```python
from build123d import *

# Parameters (mm, degrees)
SKETCH1_W           = 100
SKETCH1_H           = 45
BOSS_EXTRUDE1_DEPTH = 21
CUT_EXTRUDE1_DEPTH  = 105.629106849
CUT_EXTRUDE2_DEPTH  = 10
CUT_EXTRUDE3_DEPTH  = 57.127087934
SKETCH6_R           = 3
CUT_EXTRUDE4_DEPTH  = 56.921820428
FILLET1_R           = 4.5
SKETCH7_R           = 18
CUT_EXTRUDE5_DEPTH  = 2


with BuildPart() as part:
    # Sketch1 → Boss-Extrude1 (new body)
    with BuildSketch(Plane(origin=(0, 0, 0), x_dir=(1, 0, 0), z_dir=(0, 1, 0))):
        Rectangle(SKETCH1_W, SKETCH1_H)
    extrude(amount=BOSS_EXTRUDE1_DEPTH)

    # Sketch2 → Cut-Extrude1 (cut, through all)
    with BuildSketch(Plane(origin=(50, 0, 0), x_dir=(0, 0, -1), z_dir=(1, 0, 0))):
        Polygon((-22.5, 0), (-22.5, 5), (-15.5, 0), align=None)
        Polygon((22.5, 0), (15.5, 0), (22.5, 5), align=None)
    extrude(amount=-CUT_EXTRUDE1_DEPTH, mode=Mode.SUBTRACT)

    # Sketch3 → Cut-Extrude2 (cut)
    with BuildSketch(Plane(origin=(0, 21, 0), x_dir=(1, 0, 0), z_dir=(0, 1, 0))):
        with BuildLine():
            Line((-42, 22.5), (-42, 18))
            ThreePointArc((-42, 18), (-43.025126266, 15.525126266), (-45.5, 14.5))
            Line((-45.5, 14.5), (-50, 14.5))
            Line((-50, 14.5), (-50, 22.5))
            Line((-50, 22.5), (-42, 22.5))
        make_face()
        with BuildLine():
            Line((-50, -22.5), (-42, -22.5))
            Line((-42, -22.5), (-42, -18))
            ThreePointArc((-42, -18), (-43.025126266, -15.525126266), (-45.5, -14.5))
            Line((-45.5, -14.5), (-50, -14.5))
            Line((-50, -14.5), (-50, -22.5))
        make_face()
        with BuildLine():
            Line((42, -22.5), (42, -18))
            ThreePointArc((42, -18), (43.025126266, -15.525126266), (45.5, -14.5))
            Line((45.5, -14.5), (50, -14.5))
            Line((50, -14.5), (50, -22.5))
            Line((50, -22.5), (42, -22.5))
        make_face()
        with BuildLine():
            Line((50, 22.5), (42, 22.5))
            Line((42, 22.5), (42, 18))
            ThreePointArc((42, 18), (43.025126266, 15.525126266), (45.5, 14.5))
            Line((45.5, 14.5), (50, 14.5))
            Line((50, 14.5), (50, 22.5))
        make_face()
    extrude(amount=-CUT_EXTRUDE2_DEPTH, mode=Mode.SUBTRACT)

    # Sketch5 → Cut-Extrude3 (cut, through all)
    with BuildSketch(Plane(origin=(0, 9, 0), x_dir=(1, 0, 0), z_dir=(0, 1, 0))):
        with BuildLine():
            Line((-45.5, -14.5), (-50, -14.5))
            Line((-50, -14.5), (-50, -22.5))
            Line((-50, -22.5), (-42, -22.5))
            Line((-42, -22.5), (-42, -18))
            ThreePointArc((-42, -18), (-43.025126266, -15.525126266), (-45.5, -14.5))
        make_face()
        with BuildLine():
            Line((42, -18), (42, -22.5))
            Line((42, -22.5), (50, -22.5))
            Line((50, -22.5), (50, -14.5))
            Line((50, -14.5), (45.5, -14.5))
            ThreePointArc((45.5, -14.5), (43.025126266, -15.525126266), (42, -18))
        make_face()
        with BuildLine():
            Line((45.5, 14.5), (50, 14.5))
            Line((50, 14.5), (50, 22.5))
            Line((50, 22.5), (42, 22.5))
            Line((42, 22.5), (42, 18))
            ThreePointArc((42, 18), (43.025126266, 15.525126266), (45.5, 14.5))
        make_face()
        with BuildLine():
            Line((-42, 22.5), (-50, 22.5))
            Line((-50, 22.5), (-50, 14.5))
            Line((-50, 14.5), (-45.5, 14.5))
            ThreePointArc((-45.5, 14.5), (-43.025126266, 15.525126266), (-42, 18))
            Line((-42, 18), (-42, 22.5))
        make_face()
    extrude(amount=-CUT_EXTRUDE3_DEPTH, mode=Mode.SUBTRACT)

    # Sketch6 → Cut-Extrude4 (cut, through all)
    with BuildSketch(Plane(origin=(0, 11, 0), x_dir=(1, 0, 0), z_dir=(0, 1, 0))):
        with Locations(Location((-45.5, 18, 0), (0, 0, 270))):
            Circle(SKETCH6_R)
        with Locations(Location((-45.5, -18, 0), (0, 0, 270))):
            Circle(SKETCH6_R)
        with Locations(Location((45.5, -18, 0), (0, 0, 270))):
            Circle(SKETCH6_R)
        with Locations(Location((45.5, 18, 0), (0, 0, 270))):
            Circle(SKETCH6_R)
    extrude(amount=-CUT_EXTRUDE4_DEPTH, mode=Mode.SUBTRACT)

    # Fillet1
    fillet1_edges = [part.edges().sort_by_distance(p)[0] for p in [
        (-50, 10, 22.5),
        (50, 10, 22.5),
        (-50, 10, -22.5),
        (50, 10, -22.5),
    ]]
    fillet(fillet1_edges, radius=FILLET1_R)

    # Sketch7 → Cut-Extrude5 (cut)
    with BuildSketch(Plane(origin=(0, 21, 0), x_dir=(1, 0, 0), z_dir=(0, 1, 0))):
        with Locations(Location((-21, 0, 0), (0, 0, 270))):
            Circle(SKETCH7_R)
        with Locations(Location((21, 0, 0), (0, 0, 270))):
            Circle(SKETCH7_R)
    extrude(amount=-CUT_EXTRUDE5_DEPTH, mode=Mode.SUBTRACT)


solid = part.part
```
CAD build for the part. Positions are in the model's coordinates, mm. A direction names the side the tool comes from. Round coordinates to 2 decimals unless told otherwise and drop trailing zeros. Loops run counter-clockwise (first coordinate to the right, second up) from the corner with the lowest first, then second, coordinate; pieces in that order, holes last. Notation, with made-up numbers: M -11,-15 L 47,-15 A22 ccw 47,23 Z; hole C 56,21 d4. An arc over 180 degrees is marked long. Return JSON: item names as keys, results as strings. Group by question number.
(1) Drop flat-ended pins along their axis: P1, Ø1.3, axis at x = 47.5, y = 16, coming from the -Z side; P2, Ø5, axis at x = 47, y = 16, coming from the +Z side; P3, Ø1.3, axis at x = -48.5, y = 16.5, coming from the +Z side; P4, Ø2.5, axis at x = 47, z = 18.5, coming from the +Y side. Give the stop position or say it passes through.
(2) Saw through at A-A, the plane y = 3.25. List the corners of the cut face in (x, z), and give its area (3 significant figures).
(3) Tool access for faces 1 (the flat face through (48, 16, -14.5)), 2 (the flat face through (48, 5, -14.5)), 3 (the cylindrical face through (-31.953, 20.014, -14.284)), 4 (the flat face through (-48, 9, -20)): list every direction of +Z, -Z, +X, -X, +Y, -Y with a clear straight run to the whole face (end or side of a thin tool).
(4) Wall check: probe 1 along X at (y, z) = (10.3, 18); probe 2 along X at (y, z) = (14, 15.5); probe 3 along X at (y, z) = (2.25, 18.5). Give the ranges that are in metal, low to high. Write a range as [from, to].
(5) Saw through at B-B, the plane z = -17. List the corners of the cut face in (x, y), and give its area (3 significant figures).
(6) Saw through at D-D, the plane z = 0. List the corners of the cut face in (x, y).
(7) Mould opens along X. For faces 5 (the flat face through (42, 6, 20)), 6 (the cylindrical face through (-43.47, 10.01, 15.79)), 7 (the flat face through (0.6, 2.5, 19)) say: +X half, -X half, draft (parallel to the pull), parting line (faces both ways), or undercut.
(8) Saw through at C-C, the plane x = 21. List the corners of the cut face in (y, z), and give its area (3 significant figures).
Answer list:
{
 "1": {"P1": "z = -14.5", "P2": "z = 14.65", "P3": "z = 14.5", "P4": "through"},
 "2": {"outline": "M -50,-14.5 L -45.5,-14.5 A3.5 cw -42,-18 L -42,-20.05 L 42,-20.05 L 42,-18 A3.5 cw 45.5,-14.5 L 50,-14.5 L 50,14.5 L 45.5,14.5 A3.5 cw 42,18 L 42,20.05 L -42,20.05 L -42,18 A3.5 cw -45.5,14.5 L -50,14.5 Z", "area": "3,840 mm2"},
 "3": {"face 1": "-Z, +X, +Y", "face 2": "-Z, +X, -Y", "face 3": "+Y", "face 4": "-Z, -X, -Y"},
 "4": {"probe 1": "[-50, -48.5], [-42.5, 42.5], [48.5, 50]", "probe 2": "[-43.05, 43.05]", "probe 3": "[-42, 42]"},
 "5": {"outline": "M -50,9 L -48.33,9 L -48.33,11 L -50,11 Z; M -42.67,9 L -42.15,9 L -42.15,1.07 L 42.15,1.07 L 42.15,9 L 42.67,9 L 42.67,11 L 42.15,11 L 42.15,21 L 26.92,21 L 26.92,19 L 15.08,19 L 15.08,21 L -15.08,21 L -15.08,19 L -26.92,19 L -26.92,21 L -42.15,21 L -42.15,11 L -42.67,11 Z; M 48.33,9 L 50,9 L 50,11 L 48.33,11 Z", "area": "1,640 mm2"},
 "6": {"outline": "M -50,0 L 50,0 L 50,21 L 39,21 L 39,19 L 3,19 L 3,21 L -3,21 L -3,19 L -39,19 L -39,21 L -50,21 Z"},
 "7": {"face 5": "+X half", "face 6": "undercut", "face 7": "draft"},
 "8": {"outline": "M 0,-15.5 L 5,-22.5 L 21,-22.5 L 21,-18 L 19,-18 L 19,18 L 21,18 L 21,22.5 L 5,22.5 L 0,15.5 Z", "area": "838 mm2"}
}
